Input: part model. Units: mm. Frame: model coordinates. Coordinates: 2 decimals unless noted, no trailing zeros. One line per question, with ' | ' between items. Start each with the question number.
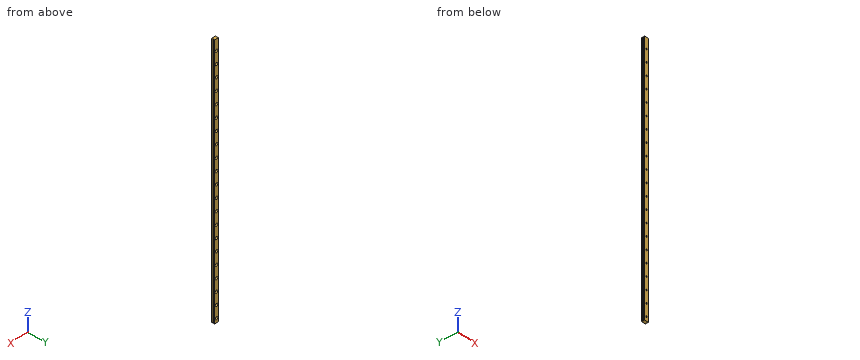
```python
from build123d import *

# Parameters (mm, degrees)
SKETCH1_W           = 5
SKETCH1_H           = 3.7
BOSS_EXTRUDE1_DEPTH = 400
SKETCH2_R           = 1.75
CUT_EXTRUDE1_DEPTH  = 2
SKETCH3_R           = 1
CUT_EXTRUDE2_DEPTH  = 401.036248358
CUT_EXTRUDE3_DEPTH  = 401.048359577
CUT_EXTRUDE_1_DEPTH = 10


with BuildPart() as part:
    # Sketch1 → Boss-Extrude1 (new body)
    with BuildSketch(Plane.XY):
        with Locations((2.5, 1.85)):
            Rectangle(SKETCH1_W, SKETCH1_H)
    extrude(amount=-BOSS_EXTRUDE1_DEPTH)

    # Sketch2 → Cut-Extrude1 (cut)
    with BuildSketch(Plane(origin=(0, 3.7, 0), x_dir=(1, 0, 0), z_dir=(0, 1, 0))):
        with Locations(Location((2.5, 5, 0), (0, 0, 270))):
            Circle(SKETCH2_R)
        with Locations(Location((2.5, 20, 0), (0, 0, 270))):
            Circle(SKETCH2_R)
        with Locations(Location((2.5, 35, 0), (0, 0, 270))):
            Circle(SKETCH2_R)
        with Locations(Location((2.5, 50, 0), (0, 0, 270))):
            Circle(SKETCH2_R)
        with Locations(Location((2.5, 65, 0), (0, 0, 270))):
            Circle(SKETCH2_R)
        with Locations(Location((2.5, 80, 0), (0, 0, 270))):
            Circle(SKETCH2_R)
        with Locations(Location((2.5, 95, 0), (0, 0, 270))):
            Circle(SKETCH2_R)
        with Locations(Location((2.5, 110, 0), (0, 0, 270))):
            Circle(SKETCH2_R)
        with Locations(Location((2.5, 125, 0), (0, 0, 270))):
            Circle(SKETCH2_R)
        with Locations(Location((2.5, 140, 0), (0, 0, 270))):
            Circle(SKETCH2_R)
        with Locations(Location((2.5, 155, 0), (0, 0, 270))):
            Circle(SKETCH2_R)
        with Locations(Location((2.5, 170, 0), (0, 0, 270))):
            Circle(SKETCH2_R)
        with Locations(Location((2.5, 185, 0), (0, 0, 270))):
            Circle(SKETCH2_R)
        with Locations(Location((2.5, 200, 0), (0, 0, 270))):
            Circle(SKETCH2_R)
        with Locations(Location((2.5, 215, 0), (0, 0, 270))):
            Circle(SKETCH2_R)
        with Locations(Location((2.5, 230, 0), (0, 0, 270))):
            Circle(SKETCH2_R)
        with Locations(Location((2.5, 245, 0), (0, 0, 270))):
            Circle(SKETCH2_R)
        with Locations(Location((2.5, 260, 0), (0, 0, 270))):
            Circle(SKETCH2_R)
        with Locations(Location((2.5, 275, 0), (0, 0, 270))):
            Circle(SKETCH2_R)
        with Locations(Location((2.5, 290, 0), (0, 0, 270))):
            Circle(SKETCH2_R)
        with Locations(Location((2.5, 305, 0), (0, 0, 270))):
            Circle(SKETCH2_R)
        with Locations(Location((2.5, 320, 0), (0, 0, 270))):
            Circle(SKETCH2_R)
        with Locations(Location((2.5, 335, 0), (0, 0, 270))):
            Circle(SKETCH2_R)
        with Locations(Location((2.5, 350, 0), (0, 0, 270))):
            Circle(SKETCH2_R)
        with Locations(Location((2.5, 365, 0), (0, 0, 270))):
            Circle(SKETCH2_R)
        with Locations(Location((2.5, 380, 0), (0, 0, 270))):
            Circle(SKETCH2_R)
        with Locations(Location((2.5, 395, 0), (0, 0, 270))):
            Circle(SKETCH2_R)
    extrude(amount=-CUT_EXTRUDE1_DEPTH, mode=Mode.SUBTRACT)

    # Sketch3 → Cut-Extrude2 (cut, through all)
    with BuildSketch(Plane(origin=(0, 1.7, 0), x_dir=(1, 0, 0), z_dir=(0, 1, 0))):
        with Locations(Location((2.5, 5, 0), (0, 0, 270))):
            Circle(SKETCH3_R)
        with Locations(Location((2.5, 20, 0), (0, 0, 270))):
            Circle(SKETCH3_R)
        with Locations(Location((2.5, 35, 0), (0, 0, 270))):
            Circle(SKETCH3_R)
        with Locations(Location((2.5, 50, 0), (0, 0, 270))):
            Circle(SKETCH3_R)
        with Locations(Location((2.5, 65, 0), (0, 0, 270))):
            Circle(SKETCH3_R)
        with Locations(Location((2.5, 80, 0), (0, 0, 270))):
            Circle(SKETCH3_R)
        with Locations(Location((2.5, 95, 0), (0, 0, 270))):
            Circle(SKETCH3_R)
        with Locations(Location((2.5, 110, 0), (0, 0, 270))):
            Circle(SKETCH3_R)
        with Locations(Location((2.5, 125, 0), (0, 0, 270))):
            Circle(SKETCH3_R)
        with Locations(Location((2.5, 140, 0), (0, 0, 270))):
            Circle(SKETCH3_R)
        with Locations(Location((2.5, 155, 0), (0, 0, 270))):
            Circle(SKETCH3_R)
        with Locations(Location((2.5, 170, 0), (0, 0, 270))):
            Circle(SKETCH3_R)
        with Locations(Location((2.5, 185, 0), (0, 0, 270))):
            Circle(SKETCH3_R)
        with Locations(Location((2.5, 200, 0), (0, 0, 270))):
            Circle(SKETCH3_R)
        with Locations(Location((2.5, 215, 0), (0, 0, 270))):
            Circle(SKETCH3_R)
        with Locations(Location((2.5, 230, 0), (0, 0, 270))):
            Circle(SKETCH3_R)
        with Locations(Location((2.5, 245, 0), (0, 0, 270))):
            Circle(SKETCH3_R)
        with Locations(Location((2.5, 260, 0), (0, 0, 270))):
            Circle(SKETCH3_R)
        with Locations(Location((2.5, 275, 0), (0, 0, 270))):
            Circle(SKETCH3_R)
        with Locations(Location((2.5, 290, 0), (0, 0, 270))):
            Circle(SKETCH3_R)
        with Locations(Location((2.5, 305, 0), (0, 0, 270))):
            Circle(SKETCH3_R)
        with Locations(Location((2.5, 320, 0), (0, 0, 270))):
            Circle(SKETCH3_R)
        with Locations(Location((2.5, 335, 0), (0, 0, 270))):
            Circle(SKETCH3_R)
        with Locations(Location((2.5, 350, 0), (0, 0, 270))):
            Circle(SKETCH3_R)
        with Locations(Location((2.5, 365, 0), (0, 0, 270))):
            Circle(SKETCH3_R)
        with Locations(Location((2.5, 380, 0), (0, 0, 270))):
            Circle(SKETCH3_R)
        with Locations(Location((2.5, 395, 0), (0, 0, 270))):
            Circle(SKETCH3_R)
    extrude(amount=-CUT_EXTRUDE2_DEPTH, mode=Mode.SUBTRACT)

    # Sketch4 → Cut-Extrude3 (cut, through all)
    with BuildSketch(Plane.XY):
        Polygon((0, 2.7), (0.5, 2.2), (0, 1.7), align=None)
        Polygon((5, 2.7), (4.5, 2.2), (5, 1.7), align=None)
    extrude(amount=-CUT_EXTRUDE3_DEPTH, mode=Mode.SUBTRACT)

    # 草图1 → 切除-拉伸1 (cut)
    with BuildSketch(Plane(origin=(0, 3.7, 0), x_dir=(1, 0, 0), z_dir=(0, 1, 0))):
        Polygon((2.5, 81.75), (15.113647071, 81.75), (15.113647071, -29.694752228), (-58.541015393, -29.694752228), (-58.541015393, 81.75), align=None)
    extrude(amount=-CUT_EXTRUDE_1_DEPTH, mode=Mode.SUBTRACT)


solid = part.part
```
(1) Material intervals for line 1 along X through (y, z) = (0.65, -245); line 2 along X through (y, z) = (2.7, -380); line 3 along Y through (x, z) = (3.2, -216.5), sorted ascending. Write a range as from..to.
(2) Pin query (flat end, axial travel): pin 1 (1 mm diameter, centred on x = 3.5, z = -125, fed in from +Y); pin 2 (1.8 mm diameter, centred on x = 2.5, z = -290, fed in from +Y). Return the tip coordinate at first contact, or that it passes through.
(3) Section A-A (y = 0.8). State how many separate pieces and enclosed holes the cut face has, then the cut area to 3 significant figures.
Worked answers:
1) line 1: x = 0..1.5, 3.5..5 | line 2: x = 0..0.75, 4.25..5 | line 3: y = 0..1.7
2) pin 1: stops at y = 1.7 | pin 2: passes through
3) separate pieces: 1 | enclosed holes: 21 | area: 1,530 mm²
